CAD build for the part. Positions are in the model's coordinates, mm. Face numbers are marked on the shaded views. A direction names the side the tool comes from. Coordinates: 2 decimals unless noted, no trailing zeros. Order: outer loops, then holes, each group sorted by start corner. A loop starts at its lowest first (then second) coordinate and runs counter-clockwise, first axis right, second up. Notation, with made-up numbers: M -23,75.25 L 3,75.25 A15 cw 3,93.25 Z; hole C 66.5,38.5 d1. An arc over 180 degrees is marked long. One line per item, written item: value.
from build123d import *

# Parameters (mm, degrees)
SKETCH_1_W          = 10
SKETCH_1_H          = 25.5
EXTRUDE_1_DEPTH     = 15
SKETCH_2_R          = 1.55
CUT_EXTRUDE_1_DEPTH = 15
SKETCH_3_R          = 3
CUT_EXTRUDE_2_DEPTH = 3
SKETCH_4_R          = 3.5
CUT_EXTRUDE_3_DEPTH = 15
SKETCH_5_W          = 8
SKETCH_5_H          = 25.5
CUT_EXTRUDE_4_DEPTH = 15
SKETCH_6_R          = 4
CUT_EXTRUDE_5_DEPTH = 2
SKETCH_7_W          = 4
SKETCH_7_H          = 5.5
CUT_EXTRUDE_6_DEPTH = 15
SKETCH_8_W          = 0.2
SKETCH_8_H          = 25.5
SKETCH_8_W_2        = 10.4
SKETCH_8_H_2        = 0.2
EXTRUDE_2_DEPTH     = 7
SKETCH_9_W          = 4
SKETCH_9_H          = 5.5
CUT_EXTRUDE_7_DEPTH = 20
SKETCH_10_W         = 1
SKETCH_10_H         = 25.7
CUT_EXTRUDE_9_DEPTH = 15
SKETCH_12_R         = 3.5
SKETCH_12_R_2       = 3.2
EXTRUDE_4_DEPTH     = 4


with BuildPart() as part:
    # 草图1 → 凸台-拉伸1 (new body)
    with BuildSketch(Plane.XY):
        with Locations((-10.315219411, -7.965383481)):
            Rectangle(SKETCH_1_W, SKETCH_1_H)
    extrude(amount=EXTRUDE_1_DEPTH)

    # 草图2 → 切除-拉伸1 (cut)
    with BuildSketch(Plane.XY.offset(15)):
        with Locations((-10.315219411, -5.715383481)):
            Circle(SKETCH_2_R)
    extrude(amount=-CUT_EXTRUDE_1_DEPTH, mode=Mode.SUBTRACT)

    # 草图3 → 切除-拉伸2 (cut)
    with BuildSketch(Plane.XY.offset(15)):
        with Locations((-10.315219411, -5.715383481)):
            Circle(SKETCH_3_R)
    extrude(amount=-CUT_EXTRUDE_2_DEPTH, mode=Mode.SUBTRACT)

    # 草图4 → 切除-拉伸3 (cut)
    with BuildSketch(Plane.XY.offset(15)):
        with Locations((-10.315219411, -16.215383481)):
            Circle(SKETCH_4_R)
    extrude(amount=-CUT_EXTRUDE_3_DEPTH, mode=Mode.SUBTRACT)

    # 草图5 → 切除-拉伸4 (cut)
    with BuildSketch(Plane(origin=(-5.315219411, 0, 0), x_dir=(0, 0, -1), z_dir=(1, 0, 0))):
        with Locations((-4, -7.965383481)):
            Rectangle(SKETCH_5_W, SKETCH_5_H)
    extrude(amount=-CUT_EXTRUDE_4_DEPTH, mode=Mode.SUBTRACT)

    # 草图6 → 切除-拉伸5 (cut)
    with BuildSketch(Plane(origin=(0, 0, 8), x_dir=(-1, 0, 0), z_dir=(0, 0, -1))):
        with Locations((10.315219411, -16.215383481)):
            Circle(SKETCH_6_R)
    extrude(amount=-CUT_EXTRUDE_5_DEPTH, mode=Mode.SUBTRACT)

    # 草图7 → 切除-拉伸6 (cut)
    with BuildSketch(Plane(origin=(-5.315219411, 0, 0), x_dir=(0, 0, -1), z_dir=(1, 0, 0))):
        with Locations((-10, 2.034616519)):
            Rectangle(SKETCH_7_W, SKETCH_7_H)
    extrude(amount=-CUT_EXTRUDE_6_DEPTH, mode=Mode.SUBTRACT)

    # 草图8 → 凸台-拉伸2 (add)
    with BuildSketch(Plane.XY.offset(15)):
        with Locations((-15.415219411, -7.965383481)):
            Rectangle(SKETCH_8_W, SKETCH_8_H)
        with Locations((-5.215219411, -7.965383481)):
            Rectangle(SKETCH_8_W, SKETCH_8_H)
        with Locations((-10.315219411, -20.815383481)):
            Rectangle(SKETCH_8_W_2, SKETCH_8_H_2)
    extrude(amount=-EXTRUDE_2_DEPTH)

    # 草图9 → 切除-拉伸7 (cut)
    with BuildSketch(Plane.ZY.offset(15.515219411)):
        with Locations((10, 2.034616519)):
            Rectangle(SKETCH_9_W, SKETCH_9_H)
    extrude(amount=-CUT_EXTRUDE_7_DEPTH, mode=Mode.SUBTRACT)

    # 草图10 → 切除-拉伸9 (cut)
    with BuildSketch(Plane.ZY.offset(15.515219411)):
        with Locations((14.5, -8.065383481)):
            Rectangle(SKETCH_10_W, SKETCH_10_H)
    extrude(amount=-CUT_EXTRUDE_9_DEPTH, mode=Mode.SUBTRACT)

    # 草图12 → 凸台-拉伸4 (add)
    with BuildSketch(Plane.XY.offset(14)):
        with Locations((-10.315219411, -16.215383481)):
            Circle(SKETCH_12_R)
        with Locations((-10.315219411, -16.215383481)):
            Circle(SKETCH_12_R_2, mode=Mode.SUBTRACT)
    extrude(amount=-EXTRUDE_4_DEPTH)


solid = part.part
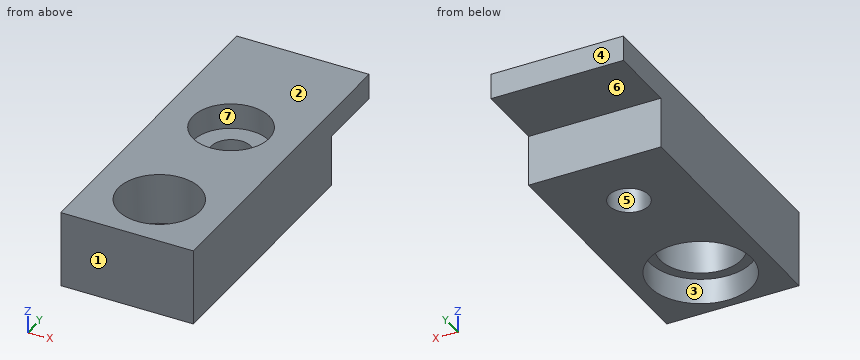
Q1. Drill centre lines: line 1 along Y through (x, z) = (-9.5, 9.45); line 2 along Y through (x, z) = (-11, 9.5); line 3 along Z through (x, y) = (-7.75, 2.25). Where is each one in solid material? Low to high.
Recorded:
line 1: y = -20.92 to -20.13, -12.3 to -7.03, -4.4 to -0.72
line 2: y = -20.92 to -20.16, -12.27 to -7.11, -4.32 to -0.72
line 3: z = 12 to 14
Q2. Slice it at A-A (y = -14.75). List the corners of the cut face in (x, z).
Recorded:
outline: M -15.52,8 L -14.04,8 L -14.04,10 L -13.16,10 L -13.16,14 L -15.52,14 Z; M -7.47,10 L -6.59,10 L -6.59,8 L -5.12,8 L -5.12,14 L -7.47,14 Z
Q3. Mould opens along Y. For the marked faces 1, 2, 3 and 4 say: released by +Y, released by -Y, zero draft, split by the parting line, or undercut.
Recorded:
face 1: released by -Y
face 2: zero draft
face 3: undercut
face 4: released by +Y
Q4. Pin check, flat tips, straight feed: pin 1 Ø4.5 at (x, y) = (-11, 2.5) entering from -Z; pin 2 Ø1.2 at (x, z) = (-13, 9.5) entering from +Y; pin 3 Ø3 at (x, y) = (-11, -6) entering from +Z. Stop position of each tip, or through.
Recorded:
pin 1: stops at z = 12
pin 2: stops at y = -0.72
pin 3: stops at z = 12
Q5. Which spindle directions (+Z, -Z, +X, -X, +Y, -Y) get a long thin tool onto all of the face, cutting with end or side? Do the marked faces 5, 6 and 7. Say none if no direction does.
Recorded:
face 5: +Z, -Z
face 6: -Z, +X, -X, +Y
face 7: +Z
Q6. Slice it at D-D (x = -6). List the corners of the cut face in (y, z).
Recorded:
outline: M -20.92,8 L -0.72,8 L -0.72,12 L 4.78,12 L 4.78,14 L -20.92,14 Z
Q7. Slice it at B-B (x = -8). List the corners of the cut face in (y, z), plus the area to 3 significant figures.
Recorded:
outline: M -20.92,8 L -19.48,8 L -19.48,10 L -18.42,10 L -18.42,14 L -20.92,14 Z; M -14.01,10 L -12.95,10 L -12.95,8 L -0.72,8 L -0.72,12 L 4.78,12 L 4.78,14 L -3.81,14 L -3.81,12 L -7.62,12 L -7.62,14 L -14.01,14 Z
area: 93.8 mm^2
Q8. Slice it at C-C (z = 12.85). List the corners of the cut face in (x, y), plus the area to 3 significant figures.
Recorded:
outline: M -15.52,-20.92 L -5.12,-20.92 L -5.12,4.78 L -15.52,4.78 Z; hole C -10.32,-16.22 d6.4; hole C -10.32,-5.72 d6
area: 207 mm^2
